Check sheet for the modelled part. Datum: model origin and axes. Units: mm. A direction names the side the tool comes from. Give positions to 0.01 mm unless a question says otherwise; leave off trailing zeros. Write each loop counter-clockwise with the first axis right and the second up, starting at its lowest first coordinate (ties: lowest second). Pieces come first, ordered by that corner, then holes. Notation, with made-up numbers: (20, -14) -> (40, -14) arc R22 ccw to (40, 2) -> close; hole circle Ø3 at (-40, 82). An arc over 180 degrees is marked (long way). Return JSON: item names as keys, results as strings.
from build123d import *


with BuildPart() as f1:
    # F0 (on Right) → F1 (revolve)
    with BuildSketch(Plane.YZ):
        with BuildLine():
            Line((-12.7, 3.175), (12.7, 3.175))
            Line((12.7, 3.175), (12.7, 10.16))
            Line((12.7, 10.16), (10.16, 11.62647))
            Line((10.16, 11.62647), (10.16, 21.39353))
            Line((10.16, 21.39353), (12.7, 22.86))
            Line((12.7, 22.86), (12.7, 42.545))
            ThreePointArc((12.7, 42.545), (11.770064, 44.790064), (9.525, 45.72))
            Line((9.525, 45.72), (-9.525, 45.72))
            ThreePointArc((-9.525, 45.72), (-11.770064, 44.790064), (-12.7, 42.545))
            Line((-12.7, 42.545), (-12.7, 22.86))
            Line((-12.7, 22.86), (-10.16, 21.39353))
            Line((-10.16, 21.39353), (-10.16, 11.62647))
            Line((-10.16, 11.62647), (-12.7, 10.16))
            Line((-12.7, 10.16), (-12.7, 3.175))
        make_face()
    revolve(axis=Axis((0, -22.93878, 0), (0, -1, 0)))


with BuildPart() as f2_1:
    # F2: copy of F1
    add(f1.part)


solid = f2_1.part
(1) Release check for a two-part mould opening along Z. For faces 4 (the cylindrical face through (3.1, 0.18, -0.69)), 5 (the conical face through (-6.4, -10.3, 20.5)), 6 (the cylindrical face through (-13.73, -0.13, 43.61)), 7 (the flat face through (18, -12.7, 18)) record: pulls with the +Z half, pulls with the -Z half, needs draft (parallel to the pull), parting line crosses it, or undercut.
Reply:
{"face 4": "undercut", "face 5": "undercut", "face 6": "parting line crosses it", "face 7": "needs draft"}
(2) Cross-section at B-B on x = 0. Enter the section's corners in (y, z) (3 decimals), then the cut area to 3 significant figures.
Reply:
{"outline": "(-12.7, -42.545) arc R3.175 ccw to (-9.525, -45.72) -> (9.525, -45.72) arc R3.175 ccw to (12.7, -42.545) -> (12.7, -22.86) -> (10.16, -21.394) -> (10.16, -11.626) -> (12.7, -10.16) -> (12.7, -3.175) -> (-12.7, -3.175) -> (-12.7, -10.16) -> (-10.16, -11.626) -> (-10.16, -21.394) -> (-12.7, -22.86) -> close; (-12.7, 3.175) -> (12.7, 3.175) -> (12.7, 10.16) -> (10.16, 11.626) -> (10.16, 21.394) -> (12.7, 22.86) -> (12.7, 42.545) arc R3.175 ccw to (9.525, 45.72) -> (-9.525, 45.72) arc R3.175 ccw to (-12.7, 42.545) -> (-12.7, 22.86) -> (-10.16, 21.394) -> (-10.16, 11.626) -> (-12.7, 10.16) -> close", "area": "2,040 mm^2"}
(3) Thickness scan on L1, parallel to X at y = 2.25, z = 0 (3 decimals); L2, parallel to Y at x = -19, z = 0.5. Record the ranges inside material, lowest first.
Reply:
{"L1": "-45.72 to -3.175, 3.175 to 45.72", "L2": "-10.16 to 10.16"}
(4) Set-up check for faces 1 (the flat face through (9, 10.16, -9)), 2 (the flat face through (18, 12.7, -18)), 3 (the flat face through (9, -10.16, 9)): record each of +Z, -Z, +X, -X, +Y, -Y from which the full face is reachable in a straight line by a thin tool's end or side.
Reply:
{"face 1": "+Y", "face 2": "+Z, -Z, +X, -X, +Y", "face 3": "-Y"}
(5) Depth check by flat-ended pin: pin 1 Ø3 at (y, z) = (8.5, -18.5) entering from +X; pin 2 Ø6 at (y, z) = (-8.5, -21) entering from -X; pin 3 Ø1.5 at (y, z) = (9, -22) entering from +X. Enter the tip coordinate at first touch or a pass-through.
Reply:
{"pin 1": "x = 42.44", "pin 2": "x = -42.03", "pin 3": "x = 40.48"}
(6) Cross-section at A-A on z = 0. Enter the section's corners in (x, y) (3 decimals).
Reply:
{"outline": "(-45.72, -9.525) arc R3.175 ccw to (-42.545, -12.7) -> (-22.86, -12.7) -> (-21.394, -10.16) -> (-11.626, -10.16) -> (-10.16, -12.7) -> (-3.175, -12.7) -> (-3.175, 12.7) -> (-10.16, 12.7) -> (-11.626, 10.16) -> (-21.394, 10.16) -> (-22.86, 12.7) -> (-42.545, 12.7) arc R3.175 ccw to (-45.72, 9.525) -> close; (3.175, -12.7) -> (10.16, -12.7) -> (11.626, -10.16) -> (21.394, -10.16) -> (22.86, -12.7) -> (42.545, -12.7) arc R3.175 ccw to (45.72, -9.525) -> (45.72, 9.525) arc R3.175 ccw to (42.545, 12.7) -> (22.86, 12.7) -> (21.394, 10.16) -> (11.626, 10.16) -> (10.16, 12.7) -> (3.175, 12.7) -> close"}
(7) Cross-section at C-C on y = -8.25. Enter the section's corners in (x, z) (3 decimals), then the cut area to 3 significant figures.
Reply:
{"outline": "circle Ø91.44 at (0, 0); hole circle Ø6.35 at (0, 0)", "area": "6,540 mm^2"}
